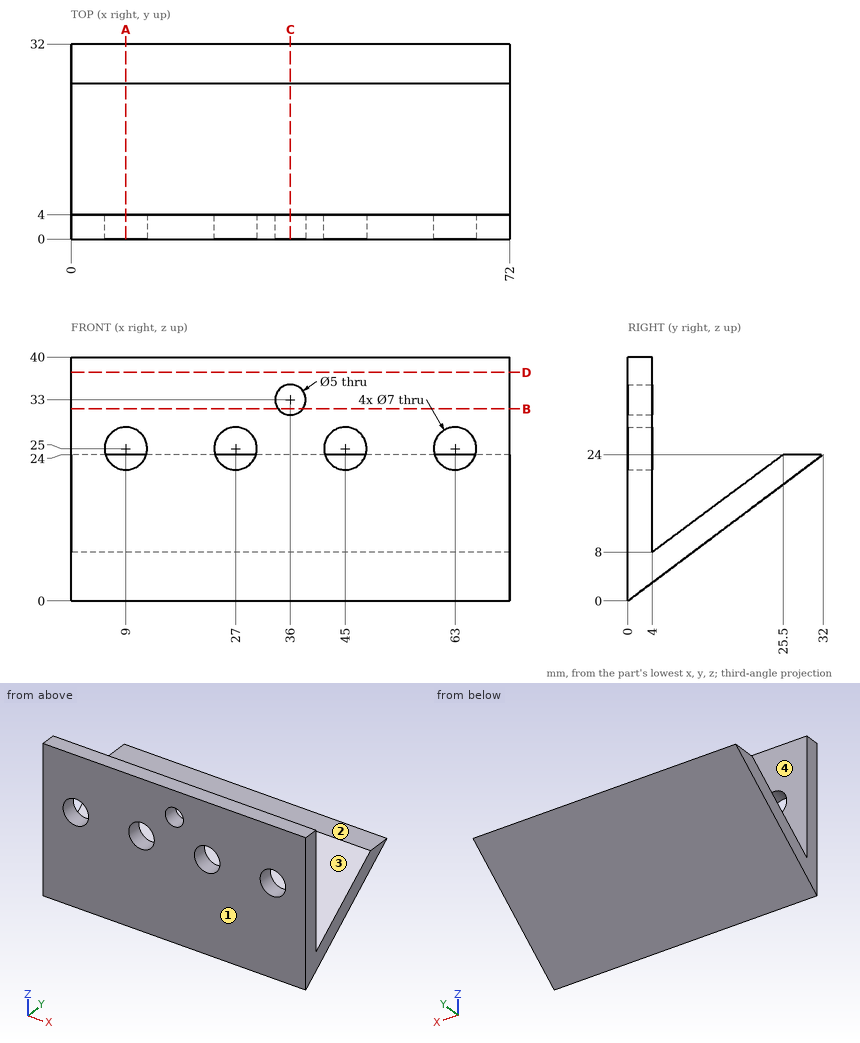
Answer from the drawing. Dimensions are ordinates in mm from the lowest x, y and z of the part. Give positions to 0.01 mm unless a question says otherwise; leave off trailing zeros. Order: outer loops, then holes, each group sorted by start corner. A loop starts at its lowest first (then second) coordinate and runs counter-clockwise, first axis right, second up.
(1) Find section A-A (x = 9). Give the vertices of the cut face in (y, z).
(2) Given pin 1 (5 mm diameter, centred on x = 24, y = 18, fed in from +Z); pin 2 (6 mm diameter, centred on x = 28.5, y = 5.5, fed in from -Z) (3 decimals); pin 3 (4 mm diameter, centred on x = 61.5, y = 25, fed in from +Z); pin 4 (4 mm diameter, centred on x = 36, z = 33, fed in from -Y), each flat-ended and moving along its own axis, determine where each tip first touches the part or whether it passes through.
(3) Straight lines are drawn through the part: L1, parallel to Y at x = 64.5, z = 12.5; L2, parallel to Z at x = 27, y = 1.45; L3, parallel to Y at x = 31, z = 21. For each, find the intervals that lie inside material, in ascending order.
(4) For a pull along Y with two mould halves and no side action, classify the marked faces 1, 2, 3 and 4 as released by +Y, released by -Y, zero draft, split by the parting line, or undercut.
(5) Find section C-C (x = 36). Give the vertices of the cut face in (y, z), plus the area to 3 significant figures.
(6) Find section B-B (z = 31.5). Give the vertices of the cut face in (x, y), plus the area to 3 significant figures.
(7) Find section D-D (z = 37.5). Give the vertices of the cut face in (x, y).
Result sheet:
1. outline: (0, 0) - (32, 24) - (25.5, 24) - (4, 8) - (4, 21.5) - (0, 21.5) - close; (0, 28.5) - (4, 28.5) - (4, 40) - (0, 40) - close
2. pin 1: stops at z = 20.28
2. pin 2: stops at z = 1.875
2. pin 3: stops at z = 24
2. pin 4: passes through
3. L1: y = 0 to 4, 10.05 to 16.67
3. L2: z = 1.09 to 21.5, 28.5 to 40
3. L3: y = 0 to 4, 21.47 to 28
4. face 1: released by -Y
4. face 2: zero draft
4. face 3: undercut
4. face 4: undercut
5. outline: (0, 0) - (32, 24) - (25.5, 24) - (4, 8) - (4, 30.5) - (0, 30.5) - close; (0, 35.5) - (4, 35.5) - (4, 40) - (0, 40) - close
5. area: 256 mm2
6. outline: (0, 0) - (34, 0) - (34, 4) - (0, 4) - close; (38, 0) - (72, 0) - (72, 4) - (38, 4) - close
6. area: 272 mm2
7. outline: (0, 0) - (72, 0) - (72, 4) - (0, 4) - close
